Input: part model. Units: mm. Frame: model coordinates. Coordinates: 2 decimals unless noted, no trailing zeros. Write each loop counter-clockwise with the first axis right and the second up, starting at its lowest first coordinate (ties: lowest second). Pieces come first, ordered by that corner, then holes. Notation, with made-up numbers: (-26, -13) - (5, -13) arc R8 ccw to (5, -1) - close; hole circle Ø10 at (69.25, 77.25). An arc over 180 degrees is marked (long way). Use a Markdown table: item, result. Add a question column.
Q1. Section query C-C (y = 1.2). Return the cut outline in (x, z) (3 decimals), then the cut area to 3 significant figures.
Q2. Material intervals for probe 1 along Y at (x, z) = (0, 0.1); probe 2 along Y at (x, z) = (-0.05, 7.5); probe 3 along Y at (x, z) = (0.25, 1), sorted ascending. Write a range as from..to.
Q3. Section query A-A (x = -1.15). Return the cut outline in (y, z) (3 decimals).
Q4. Section query B-B (z = 4.5). Return the cut outline in (x, y).
Q5. Pin query (flat end, axial travel): P1, Ø0.8, axis at x = -0.5, y = 0, coming from the +Z side; P2, Ø1.2, axis at x = 0, y = 0, coming from the +Z side (3 decimals); P3, Ø1, axis at x = 1, z = 5, coming from the -Y side. Return the tip coordinate at first contact, or that it passes through.
from build123d import *

# Parameters (mm, degrees)
F0_R     = 1.4224
F1_DEPTH = 9.525
F5_DEPTH = 0.508


with BuildPart() as f1:
    # F0 (on Top) → F1 (new body)
    with BuildSketch(Plane.XY):
        Circle(F0_R)
    extrude(amount=F1_DEPTH)

    # F2 (on Front) → F3 (revolve, cut)
    with BuildSketch(Plane.XZ):
        with BuildLine():
            Line((0, 1.524), (0, 0))
            Line((0, 0), (1.016, 0))
            Line((1.016, 0), (1.016, 0.508))
            ThreePointArc((1.016, 0.508), (0.71842, 1.22642), (0, 1.524))
        make_face()
    revolve(axis=Axis((0, 0, 0), (0, 0, -1)), mode=Mode.SUBTRACT)

    # F4 (on face) → F5 (cut)
    with BuildSketch(Plane.XY.offset(9.525)):
        Polygon((1.963537, 0.508), (0, 0.508), (-1.963537, 0.508), (-1.963537, -0.508), (0, -0.508), (1.963537, -0.508), align=None)
    extrude(amount=-F5_DEPTH, mode=Mode.SUBTRACT)


solid = f1.part
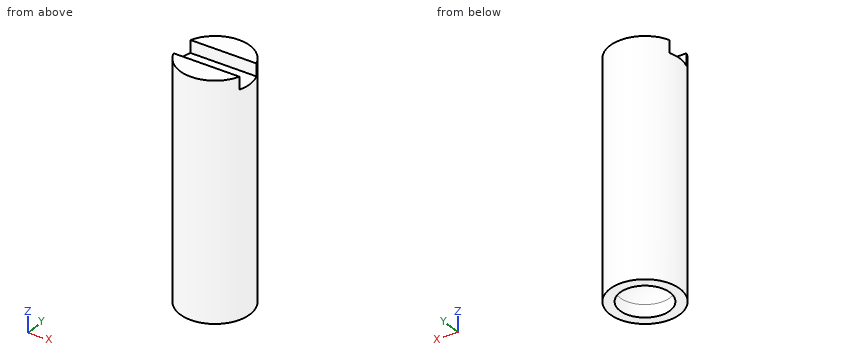
Values follow:
| question | item | result |
|---|---|---|
| 1 | outline | (-0.764, 0) - (0.764, 0) - (0.764, 9.525) - (-0.764, 9.525) - close |
| 1 | area | 14.5 mm2 |
| 2 | probe 1 | -1.42..-1.02, 1.02..1.42 |
| 2 | probe 2 | -1.42..1.42 |
| 2 | probe 3 | -1.4..-0.85, 0.85..1.4 |
| 3 | outline | (-0.837, 0) - (0.837, 0) - (0.837, 9.525) - (0.508, 9.525) - (0.508, 9.017) - (-0.508, 9.017) - (-0.508, 9.525) - (-0.837, 9.525) - close |
| 4 | outline | circle Ø2.84 at (0, 0) |
| 5 | P1 | z = 9.02 |
| 5 | P2 | z = 9.525 |
| 5 | P3 | y = -1.33 |
